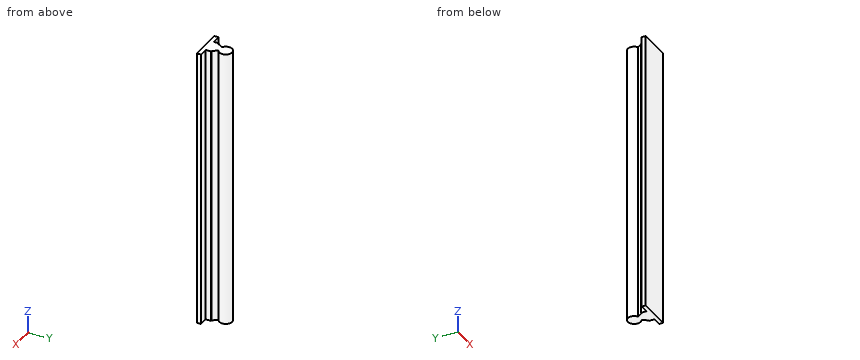
Autodesk Inventor part; units mm, degrees
ref_plane "YZ Plane" through (0, 0, 0) normal (1, 0, 0) x (0, 1, 0)
ref_plane "XZ Plane" through (0, 0, 0) normal (0, 1, 0) x (-1, 0, 0)
ref_plane "XY Plane" through (0, 0, 0) normal (0, 0, 1) x (1, 0, 0)
sketch "Sketch1" plane through (0, 0, 0) normal (0, 0, 1) x (1, 0, 0)
  line L0 (-20, 0) -> (20, 0)
  line L1 (-20, 0) -> (-20, 5)
  line L2 (20, 0) -> (20, 5)
  line L3 (-20, 5) -> (-9.25, 5)
  line L4 (20, 5) -> (9.25, 5)
  line L5 (-9.25, 5) -> (-9.25, 11.7)
  line L6 (9.25, 5) -> (9.25, 11.7)
  line L7 (-9.25, 5) -> (9.25, 5) construction
  line L8 (-9.25, 5) -> (-4.2961, 5) construction
  line L9 (9.25, 5) -> (3.3755, 5) construction
  arc A0 (4.1601, 14.485) -> (5.7961, 15.0092) centre (4, 17.8) ccw construction
  line L10 (7.926, 11.7) -> (9.25, 11.7)
  line L11 (-7.926, 11.7) -> (-9.25, 11.7)
  arc A1 (3.8717, 17.9993) -> (-3.8717, 17.9993) centre (0, 25) ccw
  line L12 (-3.8717, 17.9993) -> (-7.926, 11.7)
  line L13 (3.8717, 17.9993) -> (7.926, 11.7)
  point P0 (0, 0)
  point P1 (0, 0)
  point P2 (0, 17.8)
  point P3 (0, 5)
  point P4 (-4, 17.8)
  dimension "d0" = 40
  dimension "d1" = 5
  dimension "d2" = 5
  dimension "d3" = 10.75
  dimension "d4" = 10.75
  dimension "d5" = 6.7
  dimension "d6" = 6.7
  dimension "d15" = 25
  dimension "d16" = 18.5
  dimension "d18" = 8
extrude "Extrusion1" add sketch "Sketch1" against normal blind 350
equation "\"d1\" = d2"
equation "\"d3\" = d4"
equation "\"d5\" = d6"
properties part number "sbr16"
Source: CAD feature listing. Evaluate the final solid. Frame: model axes, mm. Coordinates: 2 decimals unless noted, no trailing zeros. Loops run counter-clockwise (first coordinate to the right, second up) from the corner with the lowest first, then second, coordinate; pieces in that order, holes last. Notation, with made-up numbers: M 43,-33 L 61,-33 A5 cw 61,-29 Z; hole C 7,45 d2. An arc over 180 degrees is marked long. Use a Markdown table: item, result. Add a question column.
Q1. Section query B-B, the plane y = 25. Return loops of the section in (x, z).
Q2. Material intervals for L1, parallel to X at y = 26.5, z = -246.5; L2, parallel to X at y = 18, z = -206.5; L3, parallel to Y at x = -13, z = -292.5, sorted ascending.
Q3. Section query A-A, the plane z = -169. Return loops of the section in (x, y), and give its area (3 significant figures).
Q4. First-contact query: pin 1 (5 mm diameter, centred on y = 24.5, z = -313, fed in from -X); pin 2 (8 mm diameter, centred on x = 7.5, y = 5, fed in from +Z); pin 3 (1.5 mm diameter, centred on x = 2, z = -147.5, fed in from +Y); pin 4 (3 mm diameter, centred on x = -13, z = -259.5, fed in from +Y). Flat tips, straight axial feed; report the tip coordinate or a pass-through.
Q5. Section query C-C, the plane x = -13. Return loops of the section in (y, z), and give its area (3 significant figures).
Result:
| question | item | result |
|---|---|---|
| 1 | outline | M -8,-350 L 8,-350 L 8,0 L -8,0 Z |
| 2 | L1 | x = -7.86 to 7.86 |
| 2 | L2 | x = -3.87 to 3.87 |
| 2 | L3 | y = 0 to 5 |
| 3 | outline | M -20,0 L 20,0 L 20,5 L 9.25,5 L 9.25,11.7 L 7.93,11.7 L 3.87,18 A8 ccw long -3.87,18 L -7.93,11.7 L -9.25,11.7 L -9.25,5 L -20,5 Z |
| 3 | area | 594 mm2 |
| 4 | pin 1 | stops at x = -8 |
| 4 | pin 2 | stops at z = 0 |
| 4 | pin 3 | stops at y = 32.9 |
| 4 | pin 4 | stops at y = 5 |
| 5 | outline | M 0,-350 L 5,-350 L 5,0 L 0,0 Z |
| 5 | area | 1,750 mm2 |
